Could you check a few things on this drawing? It's one solid part, dimensions in mm from its lowest x, y, z. A direction names the side the tool comes from. Round coordinates to 2 decimals unless told otherwise and drop trailing zeros. Write each loop counter-clockwise with the first axis right and the second up, starting at its lowest first coordinate (ties: lowest second). Pieces come first, ordered by that corner, then holes. Notation, with made-up numbers: (0.25, -35) -> (29.25, -35) arc R25 cw to (29.25, -23) -> close; hole circle Ø3 at (25.5, -9). An arc over 180 degrees is marked (long way). Return JSON: item names as keys, results as strings.
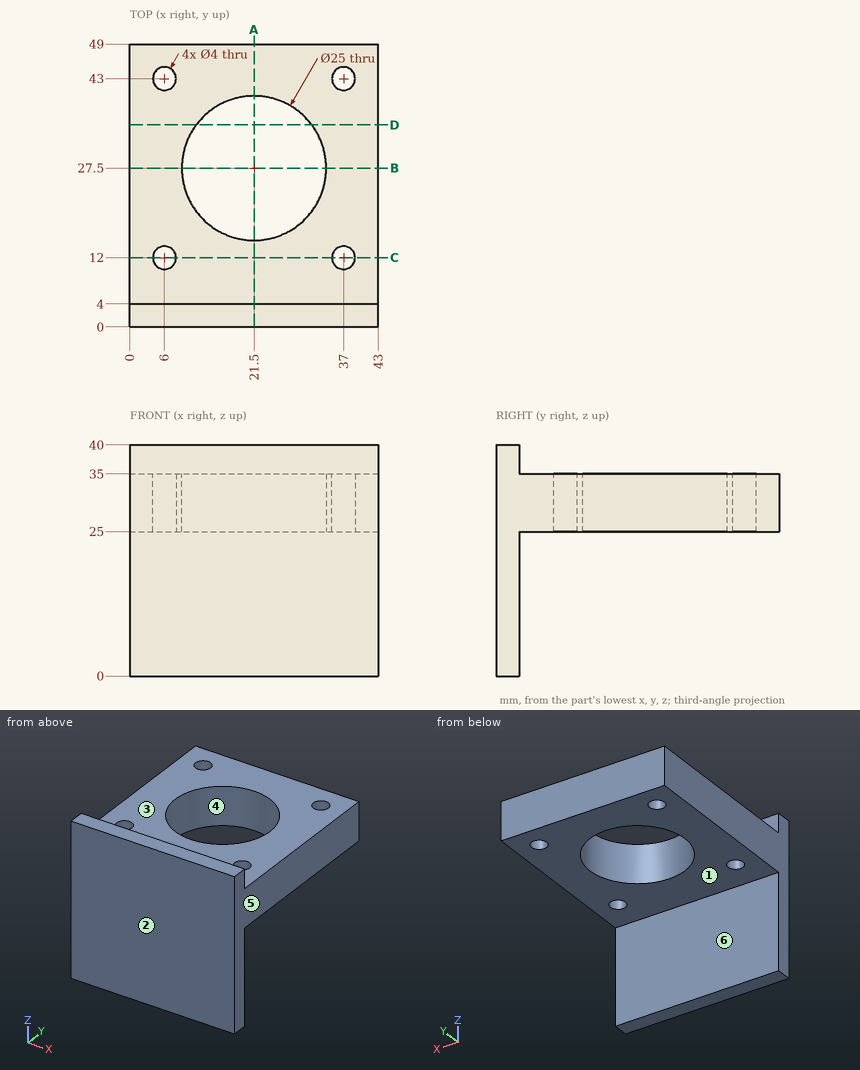
1) I want a section at B-B, the plane y = 27.5. Please give me the cut outline in (x, z), and give its area (3 significant figures).
Return value:
{"outline": "(0, 25) -> (9, 25) -> (9, 35) -> (0, 35) -> close; (34, 25) -> (43, 25) -> (43, 35) -> (34, 35) -> close", "area": "180 mm²"}
2) I want a section at A-A, the plane x = 21.5. Please give me the cut outline in (y, z), and give its area (3 significant figures).
Return value:
{"outline": "(0, 0) -> (4, 0) -> (4, 25) -> (15, 25) -> (15, 35) -> (4, 35) -> (4, 40) -> (0, 40) -> close; (40, 25) -> (49, 25) -> (49, 35) -> (40, 35) -> close", "area": "360 mm²"}
3) I want a section at C-C, the plane y = 12. Please give me the cut outline in (x, z).
Return value:
{"outline": "(0, 25) -> (4, 25) -> (4, 35) -> (0, 35) -> close; (8, 25) -> (35, 25) -> (35, 35) -> (8, 35) -> close; (39, 25) -> (43, 25) -> (43, 35) -> (39, 35) -> close"}
4) Will these pins go through, and if not, where does the flat tip stop? pin 1 Ø1.5 at (x, y) = (31, 33.5) entering from +Z; pin 2 Ø4.5 at (x, y) = (37, 43) entering from -Z; pin 3 Ø4 at (x, z) = (16, 38) entering from +Y.
Return value:
{"pin 1": "through", "pin 2": "z = 25", "pin 3": "y = 4"}
5) For the marked faces 1, 2 and 3, which set-ups out of +Z, -Z, +X, -X, +Y, -Y let a thin tool reach every point of the face, with its end or its side?
Return value:
{"face 1": "-Z, +X, -X, +Y", "face 2": "+Z, -Z, +X, -X, -Y", "face 3": "+Z, +X, -X, +Y"}
6) If I drill on probe 1 along Y at (x, z) = (37, 30.5); probe 2 along Y at (x, z) = (21, 29); probe 3 along X at (y, z) = (28, 27.5), over which ranges is the centre line in solid material (lowest first)? Write a range as [from, to].
Return value:
{"probe 1": "[0, 10], [14, 41], [45, 49]", "probe 2": "[0, 15.01], [39.99, 49]", "probe 3": "[0, 9.01], [33.99, 43]"}
7) Thinking about a two-plate mould opening in X: for the marked faces 4, 5 and 6, which applies, pulls with the +X half, pulls with the -X half, needs draft (parallel to the pull), parting line crosses it, or undercut?
Return value:
{"face 4": "undercut", "face 5": "pulls with the +X half", "face 6": "needs draft"}
8) I want a section at D-D, the plane y = 35. Please give me the cut outline in (x, z), and give its area (3 significant figures).
Return value:
{"outline": "(0, 25) -> (11.5, 25) -> (11.5, 35) -> (0, 35) -> close; (31.5, 25) -> (43, 25) -> (43, 35) -> (31.5, 35) -> close", "area": "230 mm²"}
